Here's how the part is built. I have some questions about the finished solid (model axes, mm). Coordinates: 2 decimals unless noted, no trailing zeros. Write each loop counter-clockwise with the first axis right and the second up, starting at its lowest first coordinate (ties: lowest second). Pieces come first, ordered by that corner, then holes. Notation, with made-up numbers: (86, 32) -> (126, 32) arc R11 ccw to (126, 37) -> close; hole circle Ø6 at (-4.75, -16.75). An arc over 180 degrees is marked (long way). Answer in a Markdown table with one row per item. Add a question column.
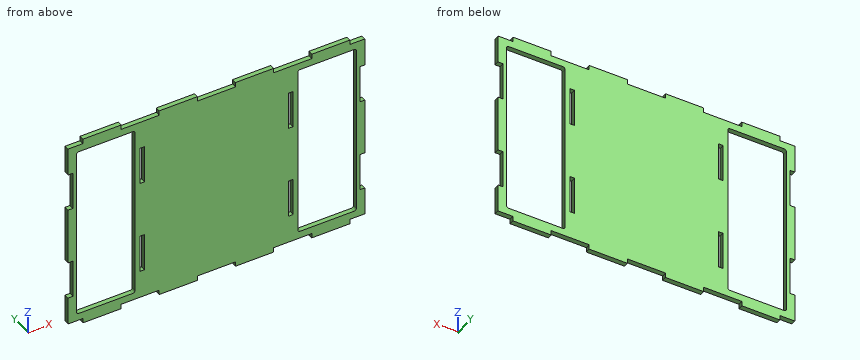
from build123d import *

# Parameters (mm, degrees)
SKETCH5_W           = 395.4
SKETCH5_H           = 265.4
BOSS_EXTRUDE3_DEPTH = 6.35
SKETCH6_W           = 78.175
SKETCH6_H           = 243.175
SKETCH6_W_2         = 75
SKETCH6_H_2         = 240
CUT_EXTRUDE1_DEPTH  = 6.35
SKETCH10_W          = 6.35
SKETCH10_H          = 50.8
SKETCH10_W_2        = 50.8
SKETCH10_H_2        = 6.35
CUT_EXTRUDE2_DEPTH  = 6.35
SKETCH11_W          = 50.8
SKETCH11_H          = 6.35
CUT_EXTRUDE3_DEPTH  = 6.35
SKETCH12_W          = 78.175
SKETCH12_H          = 4.7625
BOSS_EXTRUDE4_DEPTH = 6.35
FILLET1_R           = 3.175


with BuildPart() as part:
    # Sketch5 → Boss-Extrude3 (new body)
    with BuildSketch(Plane(origin=(0, 0, 0), x_dir=(1, 0, 0), z_dir=(0, 1, 0))):
        Rectangle(SKETCH5_W, SKETCH5_H)
    extrude(amount=BOSS_EXTRUDE3_DEPTH)

    # Sketch6 → Cut-Extrude1 (cut)
    # profile 1 of 4: a face of its own
    with BuildSketch(Plane(origin=(0, 6.35, 0), x_dir=(1, 0, 0), z_dir=(0, 1, 0))):
        with Locations((147.5, 0)):
            Rectangle(SKETCH6_W, SKETCH6_H)
        with Locations((147.5, 0)):
            Rectangle(SKETCH6_W_2, SKETCH6_H_2, mode=Mode.SUBTRACT)
    # profile 2 of 4: a face of its own
    with BuildSketch(Plane(origin=(0, 6.35, 0), x_dir=(1, 0, 0), z_dir=(0, 1, 0))):
        with Locations((147.5, 0)):
            Rectangle(SKETCH6_W_2, SKETCH6_H_2)
    # profile 3 of 4: a face of its own
    with BuildSketch(Plane(origin=(0, 6.35, 0), x_dir=(1, 0, 0), z_dir=(0, 1, 0))):
        with Locations((-147.5, 0)):
            Rectangle(SKETCH6_W, SKETCH6_H)
        with Locations((-147.5, 0)):
            Rectangle(SKETCH6_W_2, SKETCH6_H_2, mode=Mode.SUBTRACT)
    # profile 4 of 4: a face of its own
    with BuildSketch(Plane(origin=(0, 6.35, 0), x_dir=(1, 0, 0), z_dir=(0, 1, 0))):
        with Locations((-147.5, 0)):
            Rectangle(SKETCH6_W_2, SKETCH6_H_2)
    extrude(amount=-CUT_EXTRUDE1_DEPTH, mode=Mode.SUBTRACT)

    # Sketch10 → Cut-Extrude2 (cut)
    with BuildSketch(Plane.XZ):
        with Locations((98.8875, -63.5)):
            Rectangle(SKETCH10_W, SKETCH10_H)
        with Locations((98.8875, 63.5)):
            Rectangle(SKETCH10_W, SKETCH10_H)
        with Locations((-98.8875, 63.5)):
            Rectangle(SKETCH10_W, SKETCH10_H)
        with Locations((-98.8875, -63.5)):
            Rectangle(SKETCH10_W, SKETCH10_H)
        Polygon((197.7, 132.7), (177.8, 132.7), (177.8, 126.35), (191.35, 126.35), (197.7, 126.35), align=None)
        Polygon((127, 132.7), (76.2, 132.7), (76.2, 126.35), (95.7125, 126.35), (102.0625, 126.35), (108.4125, 126.35), (127, 126.35), align=None)
        with Locations((0, 129.525)):
            Rectangle(SKETCH10_W_2, SKETCH10_H_2)
        Polygon((-127, 132.7), (-127, 126.35), (-108.4125, 126.35), (-102.0625, 126.35), (-95.7125, 126.35), (-76.2, 126.35), (-76.2, 132.7), align=None)
        Polygon((-197.7, 126.35), (-191.35, 126.35), (-177.8, 126.35), (-177.8, 132.7), (-197.7, 132.7), align=None)
        Polygon((-177.8, -126.35), (-191.35, -126.35), (-197.7, -126.35), (-197.7, -132.7), (-177.8, -132.7), align=None)
        Polygon((-108.4125, -126.35), (-127, -126.35), (-127, -132.7), (-76.2, -132.7), (-76.2, -126.35), (-95.7125, -126.35), (-102.0625, -126.35), align=None)
        with Locations((0, -129.525)):
            Rectangle(SKETCH10_W_2, SKETCH10_H_2)
        Polygon((76.2, -126.35), (76.2, -132.7), (127, -132.7), (127, -126.35), (108.4125, -126.35), (102.0625, -126.35), (95.7125, -126.35), align=None)
        Polygon((177.8, -126.35), (177.8, -132.7), (197.7, -132.7), (197.7, -126.35), (191.35, -126.35), align=None)
    extrude(amount=-CUT_EXTRUDE2_DEPTH, mode=Mode.SUBTRACT)

    # Sketch11 → Cut-Extrude3 (cut)
    with BuildSketch(Plane(origin=(197.7, 0, 0), x_dir=(0, 0, -1), z_dir=(1, 0, 0))):
        with Locations((-63.5, 3.175)):
            Rectangle(SKETCH11_W, SKETCH11_H)
        with Locations((63.5, 3.175)):
            Rectangle(SKETCH11_W, SKETCH11_H)
    cut_extrude3 = extrude(amount=-CUT_EXTRUDE3_DEPTH, mode=Mode.SUBTRACT)

    # Mirror1: Cut-Extrude3 across plane
    add(cut_extrude3.mirror(Plane(origin=(0, 0, 0), x_dir=(0, 0, 1), z_dir=(1, 0, 0))), mode=Mode.SUBTRACT)

    # Sketch12 → Boss-Extrude4 (add)
    with BuildSketch(Plane.XZ):
        with Locations((147.5, -119.20625)):
            Rectangle(SKETCH12_W, SKETCH12_H)
        with Locations((147.5, 119.20625)):
            Rectangle(SKETCH12_W, SKETCH12_H)
        with Locations((-147.5, 119.20625)):
            Rectangle(SKETCH12_W, SKETCH12_H)
        with Locations((-147.5, -119.20625)):
            Rectangle(SKETCH12_W, SKETCH12_H)
    extrude(amount=-BOSS_EXTRUDE4_DEPTH)

    # Fillet1
    fillet1_edges = [part.edges().sort_by_distance(p)[0] for p in [
        (108.4125, 3.175, -116.825),
        (186.5875, 3.175, -116.825),
        (186.5875, 3.175, 116.825),
        (108.4125, 3.175, 116.825),
        (-186.5875, 3.175, 116.825),
        (-108.4125, 3.175, 116.825),
        (-108.4125, 3.175, -116.825),
        (-186.5875, 3.175, -116.825),
    ]]
    fillet(fillet1_edges, radius=FILLET1_R)


solid = part.part
Q1. Imagine slicing it at B-B on x = 133. Please give me the cut outline in (y, z) (3 decimals), plus the area to 3 significant figures.
Q2. Imagine slicing it at C-C on z = 10.5. Please give me the cut outline in (x, y).
Q3. Imagine slicing it at D-D on y = 2. State how many separate pieces and enclosed holes the cut face has, plus the area to 3 significant figures.
Q4. Imagine slicing it at A-A on z = -51.5. Please give me the cut outline in (x, y), plus the area to 3 significant figures.
Q5. I need wall thicknesses on line 1 (X direction, y = 5, z = 97); line 2 (X direction, y = 5.5, z = 44); line 3 (Z direction, x = -149, y = 1.75) (3 decimals). Which ranges of each line are inside material? Lowest first, please. Write a range as [from, to].
Q6. I'm going to push flat-ended pins straight in: P1, Ø1.9, axis at y = 4, z = 54.5, coming from the +X side; P2, Ø3, axis at x = -195, y = 3, coming from the -Z side; P3, Ø1.9, axis at y = 3.5, z = 71.5, coming from the -X side. Where does each tip first touch, or does it pass through?
Result sheet:
| question | item | result |
|---|---|---|
| 1 | outline | (0, -132.7) -> (6.35, -132.7) -> (6.35, -116.825) -> (0, -116.825) -> close; (0, 116.825) -> (6.35, 116.825) -> (6.35, 132.7) -> (0, 132.7) -> close |
| 1 | area | 202 mm^2 |
| 2 | outline | (-197.7, 0) -> (-186.59, 0) -> (-186.59, 6.35) -> (-197.7, 6.35) -> close; (-108.41, 0) -> (108.41, 0) -> (108.41, 6.35) -> (-108.41, 6.35) -> close; (186.59, 0) -> (197.7, 0) -> (197.7, 6.35) -> (186.59, 6.35) -> close |
| 3 | separate pieces | 1 |
| 3 | enclosed holes | 6 |
| 3 | area | 63,400 mm^2 |
| 4 | outline | (-191.35, 0) -> (-186.59, 0) -> (-186.59, 6.35) -> (-191.35, 6.35) -> close; (-108.41, 0) -> (-102.06, 0) -> (-102.06, 6.35) -> (-108.41, 6.35) -> close; (-95.71, 0) -> (95.71, 0) -> (95.71, 6.35) -> (-95.71, 6.35) -> close; (102.06, 0) -> (108.41, 0) -> (108.41, 6.35) -> (102.06, 6.35) -> close; (186.59, 0) -> (191.35, 0) -> (191.35, 6.35) -> (186.59, 6.35) -> close |
| 4 | area | 1,360 mm^2 |
| 5 | line 1 | x = [-197.7, -186.59], [-108.41, 108.41], [186.59, 197.7] |
| 5 | line 2 | x = [-191.35, -186.59], [-108.41, -102.06], [-95.71, 95.71], [102.06, 108.41], [186.59, 191.35] |
| 5 | line 3 | z = [-132.7, -116.825], [116.825, 132.7] |
| 6 | P1 | stops at x = 191.35 |
| 6 | P2 | stops at z = -126.35 |
| 6 | P3 | stops at x = -191.35 |
